Study the drawing (mm; zero at the part's minimum x, y, z) and answer. A direction names the side the tool comes from. Give positions to 0.01 mm unless a question says otherwise; leave off trailing zeros. Loops run counter-clockwise (first coordinate to the right, second up) from the corner with the lowest first, then second, coordinate; pieces in that order, holes last. Notation, with made-up numbers: (67, 82) -> (106, 82) arc R16 ccw to (106, 106) -> close; hole circle Ø4 at (-38, 67.25). An arc over 180 degrees is marked (long way). One line per question, with ' | ' between items. Start each with the question number.
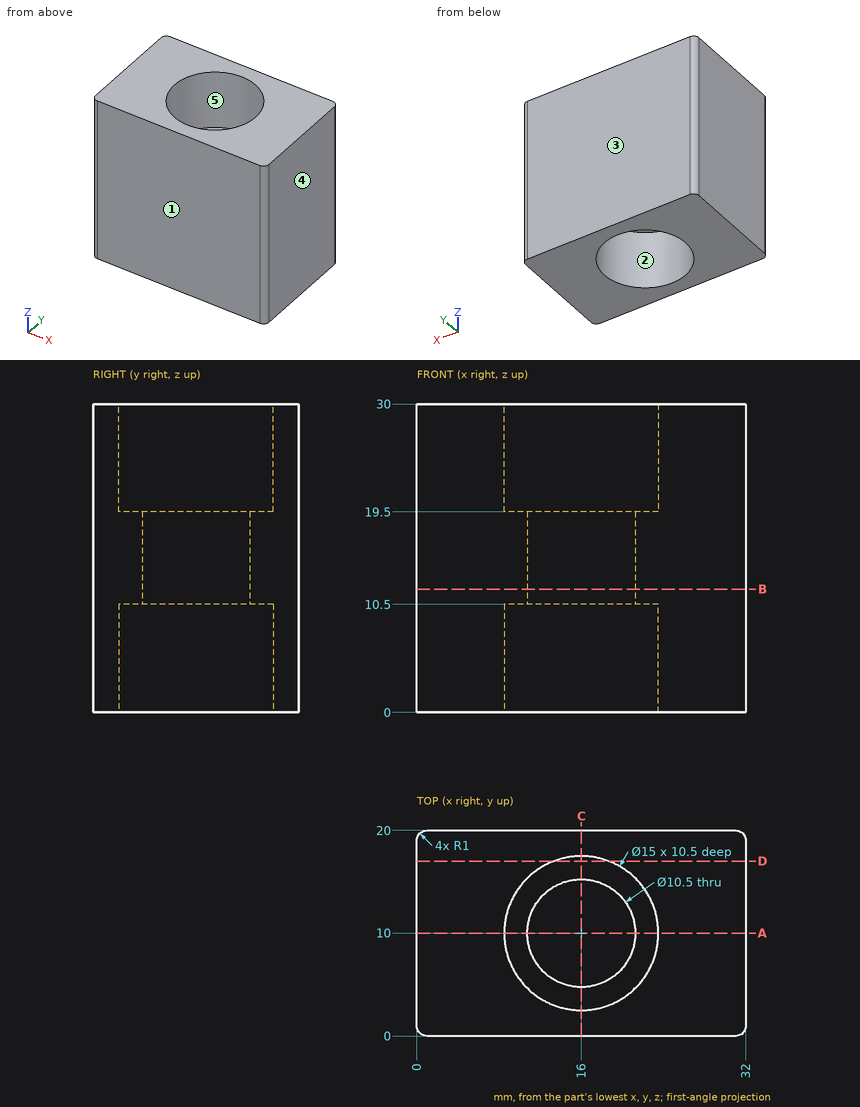
1. Each of these flat-tipped pins is pushed along its axis until it touches: pin 1 Ø8 at (x, y) = (23.5, 2.5) entering from -Z; pin 2 Ø7.5 at (x, y) = (16, 13.5) entering from -Z. Where does it stop, or does it pass through?
2. The part is cut by section B-B (z = 12). Write down the section's boundary in (x, y).
3. The part is cut by section C-C (x = 16). Write down the section's boundary in (y, z).
4. The part is cut by section A-A (y = 10). Write down the section's boundary in (x, z), plus the area to 4 significant figures.
5. Straight lines are drawn through the part: L1, parallel to X at y = 10, z = 15.5; L2, parallel to Y at x = 16, z = 17.5; L3, parallel to Y at x = 16, z = 6. For each, find the intervals that lie inside material, in ascending order.
6. Determine the mould class of the marked faces 1, 2 and 3 for opening direction Y: released by +Y, released by -Y, zero draft, split by the parting line, or undercut.
7. The part is cut by section D-D (y = 17). Write down the section's boundary in (x, z).
8. For the marked faces 4 and 5, determine the directions among +Z, -Z, +X, -X, +Y, -Y from which every point of the face is accessible in a straight line to the end or side of a thin tool.
Check sheet entries:
1) pin 1: stops at z = 0 | pin 2: stops at z = 10.5
2) outline: (0, 1) arc R1 ccw to (1, 0) -> (31, 0) arc R1 ccw to (32, 1) -> (32, 19) arc R1 ccw to (31, 20) -> (1, 20) arc R1 ccw to (0, 19) -> close; hole circle Ø10.5 at (16, 10)
3) outline: (0, 0) -> (2.5, 0) -> (2.5, 10.5) -> (4.75, 10.5) -> (4.75, 19.5) -> (2.5, 19.5) -> (2.5, 30) -> (0, 30) -> close; (15.25, 10.5) -> (17.5, 10.5) -> (17.5, 0) -> (20, 0) -> (20, 30) -> (17.5, 30) -> (17.5, 19.5) -> (15.25, 19.5) -> close
4) outline: (0, 0) -> (8.5, 0) -> (8.5, 10.5) -> (10.75, 10.5) -> (10.75, 19.5) -> (8.5, 19.5) -> (8.5, 30) -> (0, 30) -> close; (21.25, 10.5) -> (23.5, 10.5) -> (23.5, 0) -> (32, 0) -> (32, 30) -> (23.5, 30) -> (23.5, 19.5) -> (21.25, 19.5) -> close | area: 550.5 mm^2
5) L1: x = 0 to 10.75, 21.25 to 32 | L2: y = 0 to 4.75, 15.25 to 20 | L3: y = 0 to 2.5, 17.5 to 20
6) face 1: released by -Y | face 2: undercut | face 3: released by +Y
7) outline: (0, 0) -> (13.31, 0) -> (13.31, 10.5) -> (18.69, 10.5) -> (18.69, 0) -> (32, 0) -> (32, 30) -> (18.69, 30) -> (18.69, 19.5) -> (13.31, 19.5) -> (13.31, 30) -> (0, 30) -> close
8) face 4: +Z, -Z, +X, +Y, -Y | face 5: +Z
